Input: part model. Units: mm. Frame: model coordinates. A direction names the side the tool comes from. Give positions to 0.01 mm unless a question says otherwise; leave off trailing zeros. Write each loop counter-clockwise with the first axis right and the second up, starting at its lowest first coordinate (ties: lowest second). Pieces come first, ordered by that corner, then holes.
```python
from build123d import *

# Parameters (mm, degrees)
F0_W     = 482.6
F0_H     = 508
F1_DEPTH = 9.525


with BuildPart() as f1:
    # F0 (on Front) → F1 (new body)
    with BuildSketch(Plane.XZ):
        with Locations((-55.20353, 334.813255)):
            Rectangle(F0_W, F0_H)
        with BuildLine():
            ThreePointArc((135.29647, 173.523255), (123.021315, 143.888409), (93.38647, 131.613255))
            Line((93.38647, 131.613255), (-203.79353, 131.613255))
            ThreePointArc((-203.79353, 131.613255), (-233.428375, 143.888409), (-245.70353, 173.523255))
            Line((-245.70353, 173.523255), (-245.70353, 496.103255))
            ThreePointArc((-245.70353, 496.103255), (-233.428375, 525.7381), (-203.79353, 538.013255))
            Line((-203.79353, 538.013255), (93.38647, 538.013255))
            ThreePointArc((93.38647, 538.013255), (123.021315, 525.7381), (135.29647, 496.103255))
            Line((135.29647, 496.103255), (135.29647, 173.523255))
        make_face(mode=Mode.SUBTRACT)
    extrude(amount=F1_DEPTH)


with BuildPart() as f2_1:
    # F2: copy of F1
    add(f1.part.moved(Location((0, 482.6, 0))))


solid = f1.part
```
Item 1: Set-up query: faces 4 (the flat face through (156, 0, 338)), 5 (the cylindrical face through (122.694, -4.696, 526.062)). Return all of +Z, -Z, +X, -X, +Y, -Y with unobstructed straight access to the full face (end or side cutting, diameter ignored); none if empty.
Item 2: Ray query, line 1 (X direction, y = -8.75, z = 330); line 2 (Z direction, x = -65, y = -6.75); line 3 (X direction, y = -3, z = 526). Return the intervals inside material, ascending.
Item 3: Mould query, pull axis Z, two halves, no side actions, for faces 1 (the cylindrical face through (123.35, -4.7, 144.22)), 2 (the flat face through (156, -9.525, 338)), 3 (the cylindrical face through (-233.752, -4.696, 525.41)). Classes: +Z half, -Z half, draft (parallel to the pull), parting line (faces both ways), or undercut.
Item 4: Section A-A (z = 459.5). Return loops of the section in (x, y) (3 decimals), and give its area (3 significant figures).
Item 5: Section B-B (y = -4). Return loops of the section in (x, z).
Item 6: Section C-C (x = -228.5). Return loops of the section in (y, z) (3 decimals), and give its area (3 significant figures).
Solved:
1. face 4: +Z, -Z, +X, -X, +Y
1. face 5: +Y, -Y
2. line 1: x = -296.5 to -245.7, 135.3 to 186.1
2. line 2: z = 80.81 to 131.61, 538.01 to 588.81
2. line 3: x = -296.5 to -233.16, 122.76 to 186.1
3. face 1: undercut
3. face 2: draft
3. face 3: undercut
4. outline: (-296.504, -9.525) - (-245.704, -9.525) - (-245.704, 0) - (-296.504, 0) - close; (135.296, -9.525) - (186.096, -9.525) - (186.096, 0) - (135.296, 0) - close
4. area: 968 mm2
5. outline: (-296.5, 80.81) - (186.1, 80.81) - (186.1, 588.81) - (-296.5, 588.81) - close; hole (-245.7, 173.52) arc R41.91 ccw to (-203.79, 131.61) - (93.39, 131.61) arc R41.91 ccw to (135.3, 173.52) - (135.3, 496.1) arc R41.91 ccw to (93.39, 538.01) - (-203.79, 538.01) arc R41.91 ccw to (-245.7, 496.1) - close
6. outline: (-9.525, 80.813) - (0, 80.813) - (0, 139.67) - (-9.525, 139.67) - close; (-9.525, 529.956) - (0, 529.956) - (0, 588.813) - (-9.525, 588.813) - close
6. area: 1,120 mm2
